Read the model definition and answer for the solid it produces. Units are mm, in the model's axes. Face numbers are marked on the shaded views. A direction names the side the tool comes from. Give positions to 0.01 mm unless a question says otherwise; leave off trailing zeros. Order: outer loops, then holes, each group sorted by start corner. A loop starts at its lowest first (then second) coordinate and runs counter-clockwise, first axis right, second up.
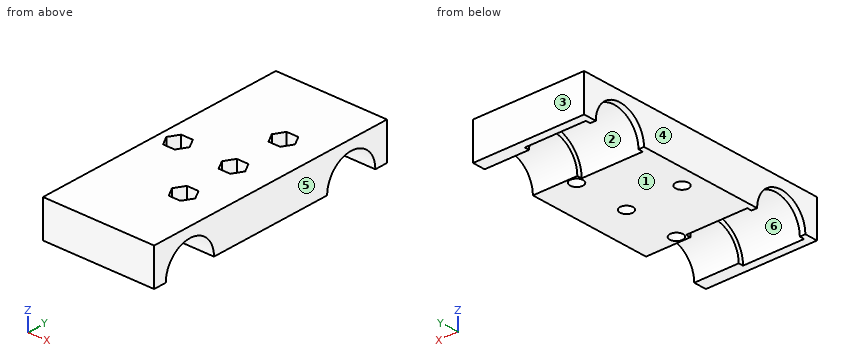
```python
from build123d import *

# Parameters (mm, degrees)
SKETCH_W        = 60
SKETCH_H        = 140
PAD_DEPTH       = 20
SKETCH001_R     = 14.5
POCKET_DEPTH    = 3
SKETCH002_R     = 17.1
POCKET001_DEPTH = 33
SKETCH003_R     = 14.5
POCKET002_DEPTH = 24.001
POCKET003_DEPTH = 6.8
SKETCH005_R     = 3.5
POCKET004_DEPTH = 13.201


with BuildPart() as part:
    # Sketch → Pad (new body)
    with BuildSketch(Plane.XY):
        with Locations((10, 0)):
            Rectangle(SKETCH_W, SKETCH_H)
    extrude(amount=PAD_DEPTH)

    # Sketch001 → Pocket (cut)
    with BuildSketch(Plane(origin=(-20, 0, 0), x_dir=(0, -1, 0), z_dir=(-1, 0, 0))):
        with Locations((-48.5, 0)):
            Circle(SKETCH001_R)
        with Locations((48.5, 0)):
            Circle(SKETCH001_R)
    extrude(amount=-POCKET_DEPTH, mode=Mode.SUBTRACT)

    # Sketch002 → Pocket001 (cut)
    with BuildSketch(Plane(origin=(-17, 0, 0), x_dir=(0, -1, 0), z_dir=(-1, 0, 0))):
        with Locations((-48.5, 0)):
            Circle(SKETCH002_R)
        with Locations((48.5, 0)):
            Circle(SKETCH002_R)
    extrude(amount=-POCKET001_DEPTH, mode=Mode.SUBTRACT)

    # Sketch003 → Pocket002 (cut, through all)
    with BuildSketch(Plane(origin=(16, 0, 0), x_dir=(0, -1, 0), z_dir=(-1, 0, 0))):
        with Locations((-48.5, 0)):
            Circle(SKETCH003_R)
        with Locations((48.5, 0)):
            Circle(SKETCH003_R)
    extrude(amount=-POCKET002_DEPTH, mode=Mode.SUBTRACT)

    # Sketch004 → Pocket003 (cut)
    with BuildSketch(Plane.XY.offset(20)):
        Polygon((-36.85, -5.45596), (-33.7, 0), (-36.85, 5.45596), (-43.15, 5.45596), (-46.3, 0), (-43.15, -5.45596), align=None)
        Polygon((23.15, 5.45596), (16.85, 5.45596), (13.7, 0), (16.85, -5.45596), (23.15, -5.45596), (26.3, 0), align=None)
        Polygon((-3.7, 0), (-6.85, 5.45596), (-13.15, 5.45596), (-16.3, 0), (-13.15, -5.45596), (-6.85, -5.45596), align=None)
        Polygon((-33.7, 30), (-36.85, 35.45596), (-43.15, 35.45596), (-46.3, 30), (-43.15, 24.54404), (-36.85, 24.54404), align=None)
        Polygon((13.7, 30), (16.85, 24.54404), (23.15, 24.54404), (26.3, 30), (23.15, 35.45596), (16.85, 35.45596), align=None)
        Polygon((-33.7, -30), (-36.85, -24.54404), (-43.15, -24.54404), (-46.3, -30), (-43.15, -35.45596), (-36.85, -35.45596), align=None)
        Polygon((13.7, -30), (16.85, -35.45596), (23.15, -35.45596), (26.3, -30), (23.15, -24.54404), (16.85, -24.54404), align=None)
    extrude(amount=-POCKET003_DEPTH, mode=Mode.SUBTRACT)

    # Sketch005 → Pocket004 (cut, through all)
    with BuildSketch(Plane.XY.offset(13.2)):
        with Locations((-40, 30)):
            Circle(SKETCH005_R)
        with Locations((20, 30)):
            Circle(SKETCH005_R)
        with Locations((20, -30)):
            Circle(SKETCH005_R)
        with Locations((-40, -30)):
            Circle(SKETCH005_R)
        with Locations((-40, 0)):
            Circle(SKETCH005_R)
        with Locations((20, 0)):
            Circle(SKETCH005_R)
        with Locations((-10, 0)):
            Circle(SKETCH005_R)
    extrude(amount=-POCKET004_DEPTH, mode=Mode.SUBTRACT)


solid = part.part
```
1) The part is cut by section A-A on x = 7. Determine the outline of the cut face in (y, z), and give its area (3 significant figures).
Final values:
outline: (-70, 0) - (-65.6, 0) arc R17.1 cw to (-31.4, 0) - (31.4, 0) arc R17.1 cw to (65.6, 0) - (70, 0) - (70, 20) - (-70, 20) - close
area: 1,880 mm2
2) The part is cut by section C-C on x = -10. Determine the outline of the cut face in (y, z), and give its area (3 significant figures).
Final values:
outline: (-70, 0) - (-65.6, 0) arc R17.1 cw to (-31.4, 0) - (-3.5, 0) - (-3.5, 13.2) - (-5.46, 13.2) - (-5.46, 20) - (-70, 20) - close; (3.5, 0) - (31.4, 0) arc R17.1 cw to (65.6, 0) - (70, 0) - (70, 20) - (5.46, 20) - (5.46, 13.2) - (3.5, 13.2) - close
area: 1,710 mm2
3) The part is cut by section B-B on z = 10.5. Count the separate pieces of the cut face and the enclosed holes in it, and give its area (3 significant figures).
Final values:
separate pieces: 3
enclosed holes: 4
area: 5,380 mm2
4) The part is cut by section D-D on y = -48.5. Determine the outline of the cut face in (x, z).
Final values:
outline: (-20, 14.5) - (-17, 14.5) - (-17, 17.1) - (16, 17.1) - (16, 14.5) - (40, 14.5) - (40, 20) - (-20, 20) - close
5) Given pin 1 (8.5 mm diameter, centred on y = -54, z = 9.5, fed in from -X); pin 2 (9 mm diameter, centred on x = 20, y = 0, fed in from +Z), each flat-ended and moving along its own axis, determine where each tip first touches the part or whether it passes through.
Final values:
pin 1: stops at x = -20
pin 2: stops at z = 13.2
6) For a pull along X with two mould halves and no side action, classify the marked faces 3, 4, 5 and 6 as released by +X, released by -X, zero draft, split by the parting line, or undercut.
Final values:
face 3: zero draft
face 4: released by -X
face 5: released by +X
face 6: undercut
7) A tool of negligible diameter and unlimited length cuts with its end or side. For the marked faces 1 and 2, from which of +Z, -Z, +X, -X, +Y, -Y can it reach the whole face along a straight path? Write none if from no direction.
Final values:
face 1: -Z, +X, -X, +Y, -Y
face 2: -Z
8) Consider L1, parallel to X at y = -51, z = 14.75; L2, parallel to Y at x = 9.5, z = 5; L3, parallel to Y at x = -1, z = 2.75. Determine where each line is inside the solid, lowest interval first.
Final values:
L1: x = -20 to -17, 16 to 40
L2: y = -70 to -64.85, -32.15 to 32.15, 64.85 to 70
L3: y = -70 to -65.38, -31.62 to 31.62, 65.38 to 70
